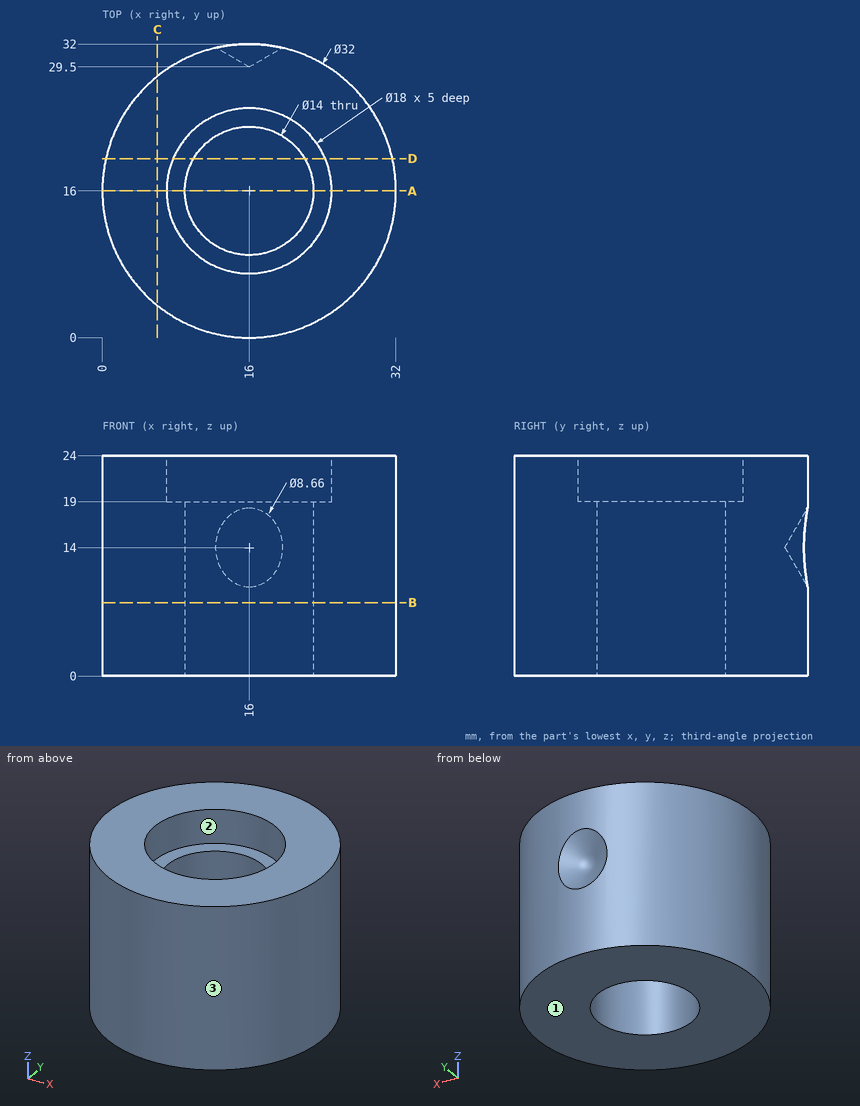
Print and shaded views of the part. All mm, measured from the part's lowest x, y and z. Coordinates: 2 decimals unless noted, no trailing zeros. Loops run counter-clockwise (first coordinate to the right, second up) from the corner with the lowest first, then second, coordinate; pieces in that order, holes last. Notation, with made-up numbers: (-38, 28) -> (5, 28) arc R15 cw to (5, 53) -> close; hole circle Ø6 at (10, 59.25). An arc over 180 degrees is marked (long way). Use a Markdown table: item, result. Add a question column.
Item 1: Band-saw the part on B-B on z = 8. Write the cut outline in (x, y), plus the area to 3 significant figures.
Item 2: Probe probe 1 along X at (y, z) = (16, 21.25); probe 2 along Z at (x, y) = (8, 18); probe 3 along X at (y, z) = (21, 20). List the from-to ranges inside material, lowest first.
Item 3: Band-saw the part on C-C on x = 6. Write the cut outline in (y, z).
Item 4: Band-saw the part on D-D on y = 19.5. Write the cut outline in (x, z).
Item 5: Pull direction X, two halves, no side cores. Call the marked faces 1, 2 and 3: +X half, -X half, draft (parallel to the pull), parting line (faces both ways), or undercut.
Item 6: Band-saw the part on A-A on y = 16. Write the cut outline in (x, z), plus the area to 3 significant figures.
Item 7: Flat gauge pins, fed straight in: P1, Ø1.5, axis at x = 26, z = 19.5, coming from the +Y side (1 decimal); P2, Ø6, axis at y = 24.5, z = 5, coming from the -X side (1 decimal); P3, Ø12, axis at y = 26.5, z = 2.5, coming from the +X side. Where does each tip first touch, or does it go through?
Geometry says:
| question | item | result |
|---|---|---|
| 1 | outline | circle Ø32 at (16, 16); hole circle Ø14 at (16, 16) |
| 1 | area | 650 mm² |
| 2 | probe 1 | 0 to 7, 25 to 32 |
| 2 | probe 2 | 0 to 19 |
| 2 | probe 3 | 0.8 to 8.52, 23.48 to 31.2 |
| 3 | outline | (3.51, 0) -> (28.49, 0) -> (28.49, 24) -> (3.51, 24) -> close |
| 4 | outline | (0.39, 0) -> (9.94, 0) -> (9.94, 19) -> (7.71, 19) -> (7.71, 24) -> (0.39, 24) -> close; (22.06, 0) -> (31.61, 0) -> (31.61, 24) -> (24.29, 24) -> (24.29, 19) -> (22.06, 19) -> close |
| 5 | face 1 | draft |
| 5 | face 2 | undercut |
| 5 | face 3 | parting line |
| 6 | outline | (0, 0) -> (9, 0) -> (9, 19) -> (7, 19) -> (7, 24) -> (0, 24) -> close; (23, 0) -> (32, 0) -> (32, 24) -> (25, 24) -> (25, 19) -> (23, 19) -> close |
| 6 | area | 412 mm² |
| 7 | P1 | y = 29.1 |
| 7 | P2 | x = 1 |
| 7 | P3 | x = 31.35 |
